Geometry: final body of the model. Coordinates: model frame, mm. Round coordinates to 2 decimals unless told otherwise and drop trailing zeros. Write each loop counter-clockwise with the first axis right and the second up, starting at its lowest first coordinate (ties: lowest second). Pieces come first, ordered by that corner, then holes.
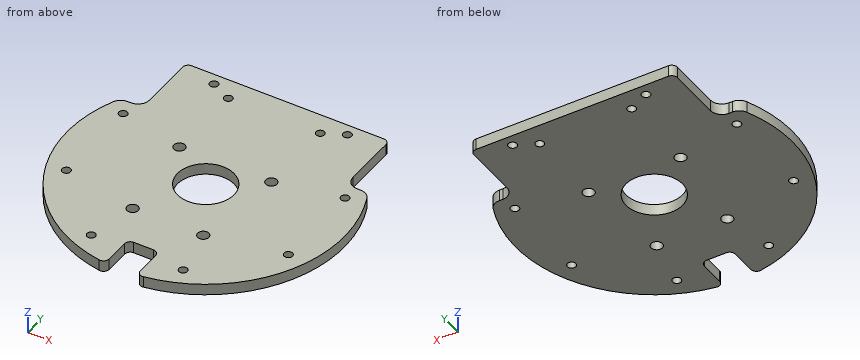
from build123d import *

# Parameters (mm, degrees)
SKETCH_1_R               = 10
SKETCH_1_R_2             = 2
SKETCH_1_R_3             = 1.5
EXTRUDE_1_DEPTH          = 4
CUT_EXTRUDE_1_DEPTH      = 69.987976837
CUT_EXTRUDE_1_DEPTH_BACK = 69.987976837
SKETCH_2_R               = 2
CUT_EXTRUDE_2_DEPTH      = 69.987976837
CUT_EXTRUDE_2_DEPTH_BACK = 69.987976837
SKETCH_3_R               = 1.5
CUT_EXTRUDE_3_DEPTH      = 69.987976837
CUT_EXTRUDE_3_DEPTH_BACK = 69.987976837
SKETCH_4_R               = 1.5


with BuildPart() as part:
    # 草图1 → 凸台-拉伸1 (new body)
    with BuildSketch(Plane.XY):
        with BuildLine():
            Line((-5.5, -46.397737014), (-5.5, -37.610257999))
            ThreePointArc((-5.5, -37.610257999), (-4.914213562, -36.196044437), (-3.5, -35.610257999))
            Line((-3.5, -35.610257999), (3.5, -35.610257999))
            ThreePointArc((3.5, -35.610257999), (4.914213562, -36.196044437), (5.5, -37.610257999))
            Line((5.5, -37.610257999), (5.5, -46.397737014))
            ThreePointArc((5.5, -46.397737014), (6.203523597, -47.920612234), (7.819148936, -48.372108802))
            ThreePointArc((7.819148936, -48.372108802), (43.01305257, -23.470775628), (44.909241811, 19.6))
            ThreePointArc((44.909241811, 19.6), (43.434071485, 21.346640106), (41.243181255, 22))
            Line((41.243181255, 22), (40, 22))
            ThreePointArc((40, 22), (37.171572875, 23.171572875), (36, 26))
            Line((36, 26), (36, 45))
            ThreePointArc((36, 45), (35.414213562, 46.414213562), (34, 47))
            Line((34, 47), (-34, 47))
            ThreePointArc((-34, 47), (-35.414213562, 46.414213562), (-36, 45))
            Line((-36, 45), (-36, 26))
            ThreePointArc((-36, 26), (-37.171572875, 23.171572875), (-40, 22))
            Line((-40, 22), (-41.243181255, 22))
            ThreePointArc((-41.243181255, 22), (-43.434071485, 21.346640106), (-44.909241811, 19.6))
            ThreePointArc((-44.909241811, 19.6), (-43.01305257, -23.470775628), (-7.819148936, -48.372108802))
            ThreePointArc((-7.819148936, -48.372108802), (-6.203523597, -47.920612234), (-5.5, -46.397737014))
        make_face()
        Circle(SKETCH_1_R, mode=Mode.SUBTRACT)
        with Locations((12.5, -21.650635095)):
            Circle(SKETCH_1_R_2, mode=Mode.SUBTRACT)
        with Locations((-12.5, -21.650635095)):
            Circle(SKETCH_1_R_2, mode=Mode.SUBTRACT)
        with Locations((-16.264045876, 39.264880132)):
            Circle(SKETCH_1_R_3, mode=Mode.SUBTRACT)
        with Locations((16.264045876, 39.264880132)):
            Circle(SKETCH_1_R_3, mode=Mode.SUBTRACT)
        with Locations((39.264880132, 16.264045876)):
            Circle(SKETCH_1_R_3, mode=Mode.SUBTRACT)
        with Locations((39.264880132, -16.264045876)):
            Circle(SKETCH_1_R_3, mode=Mode.SUBTRACT)
        with Locations((16.264045876, -39.264880132)):
            Circle(SKETCH_1_R_3, mode=Mode.SUBTRACT)
        with Locations((-16.264045876, -39.264880132)):
            Circle(SKETCH_1_R_3, mode=Mode.SUBTRACT)
        with Locations((-39.264880132, -16.264045876)):
            Circle(SKETCH_1_R_3, mode=Mode.SUBTRACT)
        with Locations((-39.264880132, 16.264045876)):
            Circle(SKETCH_1_R_3, mode=Mode.SUBTRACT)
    extrude(amount=EXTRUDE_1_DEPTH)

    # 草图2 → 切除-拉伸1 (cut, two sides: drawn at the far end of the back side and taken through both)
    with BuildSketch(Plane.XY.offset(4).offset(-CUT_EXTRUDE_1_DEPTH_BACK)):
        with Locations((-16.264045876, 11.264880132)):
            Circle(SKETCH_2_R)
        with Locations((16.264045876, 11.264880132)):
            Circle(SKETCH_2_R)
    extrude(amount=CUT_EXTRUDE_1_DEPTH + CUT_EXTRUDE_1_DEPTH_BACK, mode=Mode.SUBTRACT)

    # 草图3 → 切除-拉伸2 (cut, two sides: drawn at the far end of the back side and taken through both)
    with BuildSketch(Plane(origin=(0, 0, 0), x_dir=(-1, 0, 0), z_dir=(0, 0, -1)).offset(-CUT_EXTRUDE_2_DEPTH_BACK)):
        with Locations((-23.599902633, 42.944396943)):
            Circle(SKETCH_3_R)
    extrude(amount=CUT_EXTRUDE_2_DEPTH + CUT_EXTRUDE_2_DEPTH_BACK, mode=Mode.SUBTRACT)

    # 草图4 → 切除-拉伸3 (cut, two sides: drawn at the far end of the back side and taken through both)
    with BuildSketch(Plane(origin=(0, 0, 0), x_dir=(-1, 0, 0), z_dir=(0, 0, -1)).offset(-CUT_EXTRUDE_3_DEPTH_BACK)):
        with Locations((23.599902633, 42.944396943)):
            Circle(SKETCH_4_R)
    extrude(amount=CUT_EXTRUDE_3_DEPTH + CUT_EXTRUDE_3_DEPTH_BACK, mode=Mode.SUBTRACT)


solid = part.part
1) Line query: probe 1 along Y at (x, z) = (0, 0.95); probe 2 along Y at (x, z) = (17, 2.6); probe 3 along X at (y, z) = (-15, 3). Output: solid intervals per line, ascending.
2) First-contact query: P1, Ø2.5, axis at x = 12.5, y = -21.65, coming from the -Z side; P2, Ø2, axis at x = 13.5, z = 3.5, coming from the -Y side; P3, Ø2, axis at y = 36, z = 2, coming from the +X side. Flat tips, straight axial feed; report the tip coordinate or a pass-through.
3) Section A-A on x = 0. Output: boundary loops of the cut face in (y, z).
4) Section B-B on y = 0. Output: boundary loops of the cut face in (x, z), plus the area to 3 significant figures.
5) Section D-D on y = -13. Output: boundary loops of the cut face in (x, z).
6) Section C-C on z = 2.4. State how many separate pieces and enclosed holes the cut face has, plus the area to 3 significant figures.
Filled in:
1. probe 1: y = -35.61 to -10, 10 to 47
1. probe 2: y = -45.96 to -40.57, -37.96 to 9.41, 13.12 to 37.96, 40.57 to 47
1. probe 3: x = -46.65 to -40.07, -38.46 to 38.46, 40.07 to 46.65
2. P1: passes through
2. P2: stops at y = -47.38
2. P3: stops at x = 36
3. outline: (-35.61, 0) - (-10, 0) - (-10, 4) - (-35.61, 4) - close; (10, 0) - (47, 0) - (47, 4) - (10, 4) - close
4. outline: (-49, 0) - (-10, 0) - (-10, 4) - (-49, 4) - close; (10, 0) - (49, 0) - (49, 4) - (10, 4) - close
4. area: 312 mm2
5. outline: (-47.24, 0) - (47.24, 0) - (47.24, 4) - (-47.24, 4) - close
6. separate pieces: 1
6. enclosed holes: 15
6. area: 7,070 mm2
